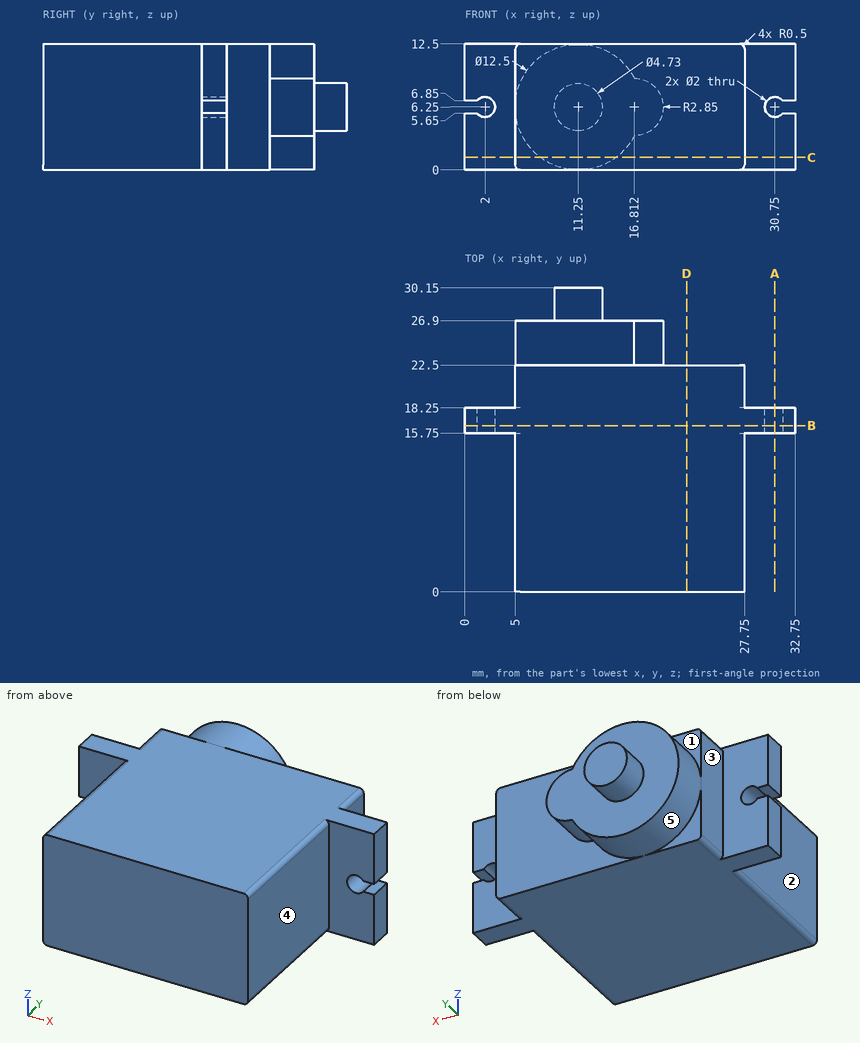
Part print with two shaded views. Sizes in mm from the minimum x, y, z corner. A direction names the side the tool comes from. Give positions to 0.01 mm unless a question says otherwise; leave off trailing zeros. Order: outer loops, then holes, each group sorted by start corner. A loop starts at its lowest first (then second) coordinate and runs counter-clockwise, first axis right, second up.
(1) Saw through at D-D, the plane x = 22. Give the cut face in (y, z).
(2) Flat gauge pins, fed straight in: pin 1 (1 mm diameter, centred on x = 15.5, z = 1.5, fed in from -Y); pin 2 (4 mm diameter, centred on x = 17.5, z = 5, fed in from +Y); pin 3 (5 mm diameter, centred on y = 10, z = 3, fed in from +X); pin 4 (6 mm diameter, centred on x = 31.5, z = 8, fed in from +Y). Where does each tip first touch, or does it go through?
(3) Saw through at B-B, the plane y = 16.5. Give the cut face in (x, z).
(4) Tool access for the marked faces 1, 2, 3, 4 and 5: list every direction of +Z, -Z, +X, -X, +Y, -Y with a clear straight run to the whole face (end or side of a thin tool).
(5) Drill centre lines: L1, parallel to Z at x = 30.75, y = 16.85; L2, parallel to X at y = 17.7, z = 6.25; L3, parallel to Y at x = 26, z = 2. Where is each one in solid material? Low to high.
(6) Saw through at A-A, the plane x = 30.75. Give the cut face in (y, z).
(7) Saw through at C-C, the plane z = 1.25. Give the cut face in (x, y).
Results found:
1. outline: (0, 0) - (22.5, 0) - (22.5, 12.5) - (0, 12.5) - close
2. pin 1: stops at y = 0
2. pin 2: stops at y = 26.9
2. pin 3: stops at x = 27.75
2. pin 4: stops at y = 18.25
3. outline: (0, 0) - (32.75, 0) - (32.75, 5.65) - (31.55, 5.65) arc R1 cw (long way) to (31.55, 6.85) - (32.75, 6.85) - (32.75, 12.5) - (0, 12.5) - (0, 6.85) - (1.2, 6.85) arc R1 cw (long way) to (1.2, 5.65) - (0, 5.65) - close
4. face 1: +Z, -X, +Y
4. face 2: +Z, -Z, -X, -Y
4. face 3: +Z, -Z, -X, +Y
4. face 4: +Z, -Z, +X, -Y
4. face 5: +Y
5. L1: z = 0 to 5.25, 7.25 to 12.5
5. L2: x = 3 to 29.75
5. L3: y = 0 to 22.5
6. outline: (15.75, 0) - (18.25, 0) - (18.25, 5.25) - (15.75, 5.25) - close; (15.75, 7.25) - (18.25, 7.25) - (18.25, 12.5) - (15.75, 12.5) - close
7. outline: (0, 15.75) - (5, 15.75) - (5, 0) - (27.75, 0) - (27.75, 15.75) - (32.75, 15.75) - (32.75, 18.25) - (27.75, 18.25) - (27.75, 22.5) - (15, 22.5) - (15, 26.9) - (7.5, 26.9) - (7.5, 22.5) - (5, 22.5) - (5, 18.25) - (0, 18.25) - close
